Input: part model. Units: mm. Frame: model coordinates. A direction names the side the tool comes from. Coordinates: 2 decimals unless noted, no trailing zeros. Loops run counter-clockwise (first coordinate to the right, second up) from the corner with the lowest first, then second, coordinate; pieces in that order, holes last. Notation, with made-up numbers: M -33,37.5 L -23,37.5 A22 cw -23,64.5 Z; hole C 59,-26.5 d2. An arc over 180 degrees is marked long. Use a Markdown table: item, result. Add a question column.
1. Section A-A on y = 0. Output: boundary loops of the cut face in (x, z).
2. Pin query (flat end, axial travel): pin 1 (0.8 mm diameter, centred on x = 5, y = 2.5, fed in from +Z); pin 2 (2 mm diameter, centred on y = -5.5, z = 5.5, fed in from -X); pin 3 (4 mm diameter, centred on x = 1, z = 1.5, fed in from -Y); pin 4 (4 mm diameter, centred on y = 3.5, z = 2.5, fed in from +X). Return the tip coordinate at first contact, or that it passes through.
3. Draft query along Y for faces 4 (the flat face through (5, 3.633, 16.558)), 5 (the flat face through (-5, -3, 19.6)), 6 (the flat face through (0.646, -6.147, 16.558)). Return one class per face: +Y half, -Y half, draft (parallel to the pull), parting line (faces both ways), or undercut.
4. Line query: L1, parallel to Y at x = 0, z = 6.75; L2, parallel to Y at x = 3.25, z = 17. Output: solid intervals per line, ascending. Write a range as [from, to].
5. Set-up query: faces 1 (the flat face through (-4.955, 3.6, 16.558)), 2 (the cylindrical face through (0, 3, 5)), 3 (the flat face through (-0.64, -6.09, 16.56)). Return all of +Z, -Z, +X, -X, +Y, -Y with unobstructed straight access to the full face (end or side cutting, diameter ignored); none if empty.
6. Section B-B on x = 0. Output: boundary loops of the cut face in (y, z).
```python
from build123d import *

# Parameters (mm, degrees)
CORTAR_REVOLUCI_N1_START = 13.6
CORTAR_REVOLUCI_N1_DEPTH = 6
MATRIZC1_COUNT           = 3
CROQUIS4_R               = 0.75
CORTAR_EXTRUIR1_DEPTH    = 31.606861976


# Read off the part's stored shape, not the designer's step: Cortar-Revolución1
with BuildPart() as part:
    # Croquis1 → Revolución1 (revolve)
    with BuildSketch(Plane.YZ):
        with BuildLine():
            Line((0, 0), (0, -9))
            ThreePointArc((0, -9), (-4.74341649, -5.58113883), (-3, 0))
            Line((-3, 0), (-3, 10))
            ThreePointArc((-3, 10), (-7.036805787, 13.954628111), (-7.291090453, 19.6))
            Line((-7.291090453, 19.6), (-4.445222154, 19.6))
            ThreePointArc((-4.445222154, 19.6), (-4.295338521, 19.444092675), (-4.45702764, 19.300465287))
            ThreePointArc((-4.45702764, 19.300465287), (-4.57485069, 19.273071665), (-4.655330258, 19.182762635))
            ThreePointArc((-4.655330258, 19.182762635), (-4.279724841, 14.326202011), (0, 12))
            Line((0, 12), (0, 0))
        make_face()
    revolve(axis=Axis((0, 0, 0), (0, 0, -1)))

    # Cortar-Revolución1 outline → Cortar-Revolución1 (cut)
    with BuildSketch(Plane.XY.offset(CORTAR_REVOLUCI_N1_START)):
        Polygon((0.945938118, -9), (0.805683263, -7.665564198), (0.387742836, -3.689126657), (0.21020847, -2), (-0.21020847, -2), (-0.387742836, -3.689126657), (-0.805683263, -7.665564198), (-0.945938118, -9), align=None)
    cortar_revoluci_n1 = extrude(amount=CORTAR_REVOLUCI_N1_DEPTH, mode=Mode.SUBTRACT)

    # MatrizC1: Cortar-Revolución1 ×3 about axis
    matrizc1_axis = Axis((0, 0, 0), (0, 0, 1))
    for i in range(1, MATRIZC1_COUNT):
        add(cortar_revoluci_n1.rotate(matrizc1_axis, i * 360 / MATRIZC1_COUNT), mode=Mode.SUBTRACT)

    # Croquis4 → Cortar-Extruir1 (cut, through all)
    with BuildSketch(Plane.XY.offset(19.6)):
        Circle(CROQUIS4_R)
    extrude(amount=-CORTAR_EXTRUIR1_DEPTH, mode=Mode.SUBTRACT)


solid = part.part
```
Answers below:
| question | item | result |
|---|---|---|
| 1 | outline | M -7.29,19.6 A7.71 ccw -3,10 L -3,0 A5 ccw -0.75,-8.94 L -0.75,12.06 A5.1 cw -4.66,19.18 A0.2 cw -4.46,19.3 A0.15 ccw long -4.45,19.6 Z; M 0.75,-8.94 A5 ccw 3,0 L 3,10 A7.71 ccw 7.29,19.6 L 4.45,19.6 A0.15 ccw long 4.46,19.3 A0.2 cw 4.66,19.18 A5.1 cw 0.75,12.06 Z |
| 2 | pin 1 | stops at z = 19.6 |
| 2 | pin 2 | passes through |
| 2 | pin 3 | stops at y = -3.48 |
| 2 | pin 4 | stops at x = 2.6 |
| 3 | face 4 | undercut |
| 3 | face 5 | draft |
| 3 | face 6 | -Y half |
| 4 | L1 | y = [-3, -0.75], [0.75, 3] |
| 4 | L2 | y = [-6.99, -3.93], [3.93, 6.99] |
| 5 | face 1 | +Z |
| 5 | face 2 | none |
| 5 | face 3 | +Z, -Y |
| 6 | outline | M -6.87,13.6 A7.71 ccw -3,10 L -3,0 A5 ccw -0.75,-8.94 L -0.75,12.06 A5.1 cw -3.71,13.6 Z; M 0.75,-8.94 A5 ccw 3,0 L 3,10 A7.71 ccw 7.29,19.6 L 4.45,19.6 A0.15 ccw long 4.46,19.3 A0.2 cw 4.66,19.18 A5.1 cw 0.75,12.06 Z |
